Geometry: final body of the model. Coordinates: model frame, mm. Face numbers are marked on the shaded views. A direction names the side the tool comes from. Give positions to 0.01 mm unless a question says otherwise; leave off trailing zeros. Loops run counter-clockwise (first coordinate to the right, second up) from the corner with the lowest first, then second, coordinate; pieces in that order, holes last. Notation, with made-up numbers: (1.25, 79) -> (48.25, 79) arc R22 cw to (48.25, 104) -> close; hole circle Ø3 at (12, -15). An arc over 180 degrees is marked (long way). One line per question, with ' | ' between items. Start each with the question number.
Item 1: Section D-D on x = -63. Return loops of the section in (y, z).
Item 2: Section B-B on z = 0. Return loops of the section in (x, y).
Item 3: Section A-A on x = 0. Return loops of the section in (y, z).
Item 4: Material intervals for line 1 along X through (y, z) = (1.5, 240); line 2 along X through (y, z) = (2.25, 38.5); line 3 along Y through (x, z) = (25.5, 0), sorted ascending. Write a range as [from, to].
Item 5: Set-up query: the marked faces 1 and 2. Return all of +Z, -Z, +X, -X, +Y, -Y with unobstructed straight access to the full face (end or side cutting, diameter ignored); none if empty.
Item 6: Section C-C on y = 0. Give the number of separate pieces and of enclosed holes in the cut face, then the cut area to 3 significant figures.
Item 7: Pin query (flat end, axial travel): P1, Ø10, axis at x = 18.5, y = -8, coming from the -Z side; P2, Ø5, axis at y = 1.5, z = 41, coming from the -X side; P3, Ø8, axis at y = -0.5, z = 81, coming from the +X side. Return the tip coordinate at first contact, or that it passes through.
from build123d import *

# Parameters (mm, degrees)
SKETCH_1_R      = 15
SKETCH_1_R_2    = 7.5
EXTRUDE_1_DEPTH = 75
SKETCH_2_R      = 12.5
EXTRUDE_2_DEPTH = 5
FILLET_1_R      = 4
FILLET_2_R      = 20
FILLET_3_R      = 2


with BuildPart() as part:
    # 스케치1 → 보스-돌출1 (new, symmetric)
    with BuildSketch(Plane(origin=(0, 0, 0), x_dir=(0, 0, -1), z_dir=(1, 0, 0))):
        Circle(SKETCH_1_R)
        Circle(SKETCH_1_R_2, mode=Mode.SUBTRACT)
    extrude(amount=EXTRUDE_1_DEPTH, both=True)

    # 스케치2 → 보스-돌출2 (add, symmetric)
    with BuildSketch(Plane(origin=(0, 0, 0), x_dir=(1, 0, 0), z_dir=(0, 1, 0))):
        with BuildLine():
            Line((-70, -65), (-25, -215))
            Line((-25, -215), (-25, -240))
            ThreePointArc((-25, -240), (0, -265), (25, -240))
            Line((25, -240), (25, -215))
            Line((25, -215), (70, -65))
            Line((70, -65), (70, -12))
            Line((70, -12), (45, -12))
            Line((45, -12), (45, -61.330779092))
            Line((45, -61.330779092), (36.399233728, -90))
            Line((36.399233728, -90), (-36.399233728, -90))
            Line((-36.399233728, -90), (-45, -61.330779092))
            Line((-45, -61.330779092), (-45, -12))
            Line((-45, -12), (-70, -12))
            Line((-70, -12), (-70, -65))
        make_face()
        with Locations(Location((0, -240, 0), (0, 0, 270))):
            Circle(SKETCH_2_R, mode=Mode.SUBTRACT)
        with BuildLine():
            Line((3.831305141, -198.559761956), (28.899233728, -115))
            Line((28.899233728, -115), (-28.899233728, -115))
            Line((-28.899233728, -115), (-3.831305141, -198.559761956))
            ThreePointArc((-3.831305141, -198.559761956), (0, -201.410370414), (3.831305141, -198.559761956))
        make_face(mode=Mode.SUBTRACT)
    extrude(amount=EXTRUDE_2_DEPTH, both=True)

    # 필렛1
    fillet_1_edges = [part.edges().sort_by_distance(p)[0] for p in [
        (36.399233728, 0, 90),
        (-36.399233728, 0, 90),
        (28.899233728, 0, 115),
        (-28.899233728, 0, 115),
    ]]
    fillet(fillet_1_edges, radius=FILLET_1_R)

    # 필렛2
    fillet_2_edges = [part.edges().sort_by_distance(p)[0] for p in [
        (-70, 0, 65),
        (70, 0, 65),
        (45, 0, 61.330779092),
        (-45, 0, 61.330779092),
    ]]
    fillet(fillet_2_edges, radius=FILLET_2_R)

    # 필렛3
    fillet_3_edges = [part.edges().sort_by_distance(p)[0] for p in [
        (-45, 0, 15),
        (-57.5, -5, 14.142135624),
        (-57.5, 5, 14.142135624),
        (-70, 0, 15),
        (45, 0, 15),
        (57.5, -5, 14.142135624),
        (57.5, 5, 14.142135624),
        (70, 0, 15),
    ]]
    fillet(fillet_3_edges, radius=FILLET_3_R)


solid = part.part
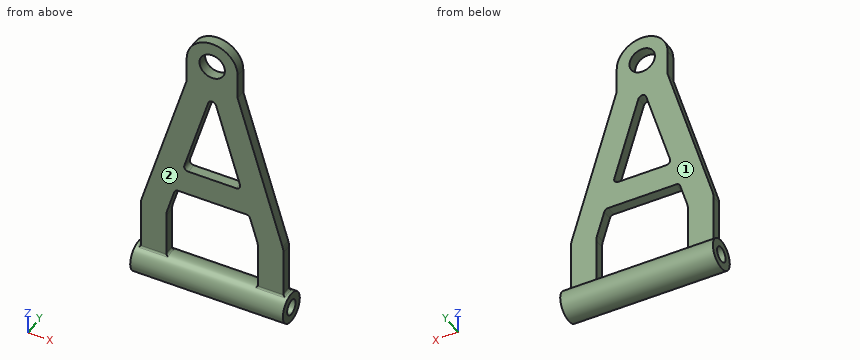
Result sheet:
1) outline: (-6.18, 13.67) arc R15 ccw (long way) to (6.18, 13.67) arc R2 cw to (5, 15.49) -> (5, 88.33) -> (-5, 88.33) -> (-5, 15.49) arc R2 cw to start; hole circle Ø15 at (0, 0)
2) outline: (-75, -15) -> (75, -15) -> (75, -7.5) -> (-75, -7.5) -> close; (-75, 7.5) -> (75, 7.5) -> (75, 15) -> (-75, 15) -> close
3) outline: circle Ø30 at (0, 0); (-5, 90) -> (5, 90) -> (5, 115) -> (-5, 115) -> close; (-5, 201.41) -> (5, 201.41) -> (5, 227.5) -> (-5, 227.5) -> close; (-5, 252.5) -> (5, 252.5) -> (5, 265) -> (-5, 265) -> close; hole circle Ø15 at (0, 0)
4) line 1: x = [-25, -12.5], [12.5, 25] | line 2: x = [-70, -45], [45, 70] | line 3: y = [-15, -7.5], [7.5, 15]
5) face 1: +Z, +X, -X, +Y | face 2: +Z, +X, -X, -Y
6) separate pieces: 2 | enclosed holes: 3 | area: 16,000 mm²
7) P1: stops at z = -14.7 | P2: stops at x = -70 | P3: stops at x = 66.4
